```python
from build123d import *
from build123d.topology import SkipClean

# Parameters (mm, degrees)
SKETCH1_R                = 2.4
BOSS_EXTRUDE1_DEPTH      = 5
BOSS_EXTRUDE2_DEPTH      = 3
BOSS_EXTRUDE2_DEPTH_BACK = 8
SKETCH3_R                = 2.4
CUT_EXTRUDE1_DEPTH       = 2.5
CUT_EXTRUDE1_DEPTH_BACK  = 2.5
SKETCH4_R                = 2.4
FILLET1_R                = 30
SCALE1_SCALE             = 0.8
CUT_EXTRUDE2_DEPTH       = 49.577813504
CUT_EXTRUDE2_DEPTH_BACK  = 49.577813504
SKETCH5_R                = 2
FILLET2_R                = 1
FILLET3_R                = 10


with BuildPart() as part:
    # Sketch1 → Boss-Extrude1 (new body)
    with BuildSketch(Plane(origin=(0, 0, 0), x_dir=(1, 0, 0), z_dir=(0, 1, 0))):
        with BuildLine():
            Line((-51.5565916, 7.5), (51.5565916, 7.5))
            ThreePointArc((51.5565916, 7.5), (59.0565916, 0), (51.5565916, -7.5))
            Line((51.5565916, -7.5), (-51.5565916, -7.5))
            ThreePointArc((-51.5565916, -7.5), (-59.0565916, 0), (-51.5565916, 7.5))
        make_face()
        with Locations(Location((-51.5565916, 0, 0), (0, 0, 270))):
            Circle(SKETCH1_R, mode=Mode.SUBTRACT)
        with Locations(Location((51.5565916, 0, 0), (0, 0, 270))):
            Circle(SKETCH1_R, mode=Mode.SUBTRACT)
    extrude(amount=BOSS_EXTRUDE1_DEPTH)

    # Sketch3 → Boss-Extrude2 (add, two sides: drawn at the far end of the back side and taken through both)
    with SkipClean():  # the faces are left unmerged after this step: merging them gives an invalid solid
        with BuildSketch(Plane(origin=(0, 5, 0), x_dir=(1, 0, 0), z_dir=(0, 1, 0)).offset(-BOSS_EXTRUDE2_DEPTH_BACK)):
            with BuildLine():
                Line((51.5565916, 7.5), (39.5565916, 7.5))
                Line((39.5565916, 7.5), (39.5565916, -7.5))
                Line((39.5565916, -7.5), (51.5565916, -7.5))
                ThreePointArc((51.5565916, -7.5), (59.0565916, 0), (51.5565916, 7.5))
            make_face()
            with Locations(Location((51.5565916, 0, 0), (0, 0, 270))):
                Circle(SKETCH3_R, mode=Mode.SUBTRACT)
        extrude(amount=BOSS_EXTRUDE2_DEPTH + BOSS_EXTRUDE2_DEPTH_BACK)
    add(part.part.scale(1), mode=Mode.REPLACE)  # the faces are merged on a copy

    # Sketch4 → Cut-Extrude1 (cut, two sides: drawn at the far end of the back side and taken through both)
    with BuildSketch(Plane(origin=(0, 2.5, 0), x_dir=(1, 0, 0), z_dir=(0, 1, 0)).offset(-CUT_EXTRUDE1_DEPTH_BACK)):
        with BuildLine():
            Line((42.5565916, 7.5), (42.5565916, -7.5))
            Line((42.5565916, -7.5), (51.5565916, -7.5))
            ThreePointArc((51.5565916, -7.5), (59.0565916, 0), (51.5565916, 7.5))
            Line((51.5565916, 7.5), (42.5565916, 7.5))
        make_face()
        with Locations(Location((51.5565916, 0, 0), (0, 0, 270))):
            Circle(SKETCH4_R, mode=Mode.SUBTRACT)
    extrude(amount=CUT_EXTRUDE1_DEPTH + CUT_EXTRUDE1_DEPTH_BACK, mode=Mode.SUBTRACT)

    # Fillet1
    # the kernel refuses this fillet: 30 mm, written as the material it adds along each edge
    with BuildSketch(Plane(origin=(39.5565916, 0, -7.5), x_dir=(0, -1, 0), z_dir=(0, 0, 1))) as fillet1_piece_1:
        with BuildLine():
            CenterArc((30, -13.076696831), FILLET1_R, 154.158067237, 25.841932763)
            Line((0, -13.076696831), (-0.6, -13.076696831))
            Line((-0.6, -13.076696831), (-0.6, 0))
            Line((-0.6, 0), (0, 0.6))
            ThreePointArc((0, 0.6), (1.5, 0.6), (2.46, 0.261533937))
            Line((2.46, 0.261533937), (3, 0))
        make_face()
    extrude(amount=15)
    with BuildSketch(Plane(origin=(39.5565916, 5, -7.5), x_dir=(-1, 0, 0), z_dir=(0, 0, 1))) as fillet1_piece_2:
        with BuildLine():
            CenterArc((13.076696831, -30), FILLET1_R, 90, 25.841932763)
            Line((0, -3), (-0.261533937, -2.46))
            ThreePointArc((-0.261533937, -2.46), (-0.6, -1.5), (-0.6, 0))
            Line((-0.6, 0), (0, 0.6))
            Line((0, 0.6), (13.076696831, 0.6))
            Line((13.076696831, 0.6), (13.076696831, 0))
        make_face()
    extrude(amount=15)


with BuildPart() as part_1:
    # Scale1: scaled about (3.796755654, 2.5, 0)
    add(part.part.scale(SCALE1_SCALE).moved(Location((0.759351131, 0.5, 0))))

    # Sketch5 → Cut-Extrude2 (cut, two sides: drawn at the far end of the back side and taken through both)
    with BuildSketch(Plane(origin=(0, 2.5, 0), x_dir=(1, 0, 0), z_dir=(0, 1, 0)).offset(-CUT_EXTRUDE2_DEPTH_BACK)):
        with Locations(Location((-40.485922149, 0, 0), (0, 0, 270))):
            Circle(SKETCH5_R)
        with Locations(Location((42.004624411, 0, 0), (0, 0, 270))):
            Circle(SKETCH5_R)
    extrude(amount=CUT_EXTRUDE2_DEPTH + CUT_EXTRUDE2_DEPTH_BACK, mode=Mode.SUBTRACT)

    # Fillet2
    fillet2_edges = [part_1.edges().sort_by_distance(p)[0] for p in [
        (34.804624411, 4.5, 0),
        (34.804624411, 0.5, 0),
    ]]
    fillet(fillet2_edges, radius=FILLET2_R)

    # Fillet3
    fillet3_edges = [part_1.edges().sort_by_distance(p)[0] for p in [
        (32.404624411, -1.9, 0),
        (32.404624411, 6.9, 0),
    ]]
    fillet(fillet3_edges, radius=FILLET3_R)


solid = part_1.part
```
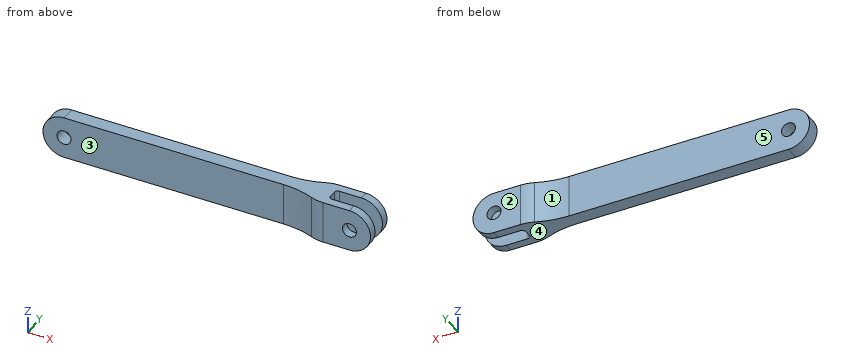
The model under review builds one solid part; all positions refer to its coordinate system, in mm. Face numbers are marked on the shaded views. A direction names the side the tool comes from. Coordinates: 2 decimals unless noted, no trailing zeros. Loops run counter-clockwise (first coordinate to the right, second up) from the corner with the lowest first, then second, coordinate; pieces in that order, holes last. Notation, with made-up numbers: (75.5, -10.75) -> (109.5, -10.75) arc R15 ccw to (109.5, 12.25) -> close; hole circle Ø7 at (28, 58.25). An arc over 180 degrees is marked (long way). Answer as CSV lines item,"result".
Item 1: Draft analysis for pull direction X (two halves, no side actions). For the marked faces 1 and 2, state which applies: +X half, -X half, draft (parallel to the pull), parting line (faces both ways), or undercut.
Results below:
face 1,"-X half"
face 2,"draft"
Item 2: Take a section at A-A, the plane z = 0. State the section outline as (x, y) points.
Results below:
outline,"(-46.49, 0.5) -> (-42.49, 0.5) -> (-42.49, 4.5) -> (-46.49, 4.5) -> close; (-38.49, 0.5) -> (21.94, 0.5) arc R24 cw to (30.8, -1.19) arc R10 ccw to (34.49, -1.9) -> (40, -1.9) -> (40, 0.5) -> (35.8, 0.5) arc R1 cw to (34.8, 1.5) -> (34.8, 3.5) arc R1 cw to (35.8, 4.5) -> (40, 4.5) -> (40, 6.9) -> (34.49, 6.9) arc R10 ccw to (30.8, 6.19) arc R24 cw to (21.94, 4.5) -> (-38.49, 4.5) -> close; (44, -1.9) -> (48, -1.9) -> (48, 0.5) -> (44, 0.5) -> close; (44, 4.5) -> (48, 4.5) -> (48, 6.9) -> (44, 6.9) -> close"
Item 3: Insertion check: pin 1 (2 mm diameter, centred on y = 4, z = -3.5, fed in from +X); pin 2 (1 mm diameter, centred on y = 2, z = -1.5, fed in from +X); pin 3 (5 mm diameter, centred on x = -40.49, z = 0, fed in from +Y); pin 4 (6.5 mm diameter, centred on x = 42, z = 0, fed in from -Y). Each pin has a flat end and moves straight along its axis. Give the tip position at first contact, or say it passes through.
Results below:
pin 1,"stops at x = 47.4"
pin 2,"stops at x = 34.8"
pin 3,"stops at y = 4.5"
pin 4,"stops at y = -1.9"
Item 4: Take a section at C-C, the plane x = 10. State the section outline as (y, z) points, and give its area (3 significant figures).
Results below:
outline,"(0.5, -6) -> (4.5, -6) -> (4.5, 6) -> (0.5, 6) -> close"
area,"48.0 mm2"
Item 5: For L1, parallel to Y at x = 43, z = 3; L2, parallel to Y at x = -14.5, z = -2.75; L3, parallel to X at y = 4, z = -0.5, list the stretches that pass through material, from the lowest coordinate up.
Results below:
L1,"y = -1.9 to 0.5, 4.5 to 6.9"
L2,"y = 0.5 to 4.5"
L3,"x = -46.47 to -42.42, -38.55 to 34.94"
Item 6: Take a section at B-B, the plane z = 3.75. State the section outline as (x, y) points, and give its area (3 significant figures).
Results below:
outline,"(-45.17, 0.5) -> (21.94, 0.5) arc R24 cw to (30.8, -1.19) arc R10 ccw to (34.49, -1.9) -> (46.69, -1.9) -> (46.69, 0.5) -> (35.8, 0.5) arc R1 cw to (34.8, 1.5) -> (34.8, 3.5) arc R1 cw to (35.8, 4.5) -> (46.69, 4.5) -> (46.69, 6.9) -> (34.49, 6.9) arc R10 ccw to (30.8, 6.19) arc R24 cw to (21.94, 4.5) -> (-45.17, 4.5) -> close"
area,"405 mm2"
Item 7: Machinability: for the marked faces 3, 4 and 5, which of the approach directions +Z, -Z, +X, -X, +Y, -Y give a long, thin tool a straight path to every point of the face, cutting with its end or side? Answer none if there is none.
Results below:
face 3,"+Z, -Z, -X, -Y"
face 4,"-Z, +X, -X, +Y, -Y"
face 5,"+Z, -Z, -X, +Y"
